The listing builds one solid part. Answer for the finished solid, in the listing's coordinates (mm). A direction names the side the tool comes from. Give positions to 0.01 mm unless a question says otherwise; leave off trailing zeros. Write each loop counter-clockwise with the first axis right and the second up, starting at its lowest first coordinate (ties: lowest second). Pieces come first, ordered by that corner, then holes. Notation, with made-up numbers: (-0.75, -16) - (40.25, -16) arc R17 ccw to (40.25, -5) - close; hole circle Ø10 at (82.5, 51). An arc over 180 degrees is marked (long way). Return JSON: item names as keys, results as strings.
from build123d import *

# Parameters (mm, degrees)
SKETCH1_W           = 160
SKETCH1_H           = 102
SKETCH1_W_2         = 154
SKETCH1_H_2         = 96
BOSS_EXTRUDE1_DEPTH = 40
SKETCH2_W           = 160
SKETCH2_H           = 102
BOSS_EXTRUDE2_DEPTH = 3
SKETCH3_R           = 1.5
BOSS_EXTRUDE3_DEPTH = 3


with BuildPart() as part:
    # Sketch1 → Boss-Extrude1 (new body)
    with BuildSketch(Plane(origin=(0, 0, 0), x_dir=(1, 0, 0), z_dir=(0, 1, 0))):
        with Locations((77, -48)):
            Rectangle(SKETCH1_W, SKETCH1_H)
        with Locations((77, -48)):
            Rectangle(SKETCH1_W_2, SKETCH1_H_2, mode=Mode.SUBTRACT)
    extrude(amount=BOSS_EXTRUDE1_DEPTH)

    # Sketch2 → Boss-Extrude2 (add)
    with BuildSketch(Plane.XZ):
        with Locations((77, 48)):
            Rectangle(SKETCH2_W, SKETCH2_H)
    extrude(amount=BOSS_EXTRUDE2_DEPTH)

    # Sketch3 → Boss-Extrude3 (add)
    with BuildSketch(Plane.XZ.offset(3)):
        with BuildLine():
            Line((87, 103), (87, -7))
            ThreePointArc((87, -7), (77, -17), (67, -7))
            Line((67, -7), (67, 103))
            ThreePointArc((67, 103), (77, 113), (87, 103))
        make_face()
        with Locations(Location((77, -7, 0), (0, 0, 270))):
            Circle(SKETCH3_R, mode=Mode.SUBTRACT)
        with Locations(Location((77, 103, 0), (0, 0, 270))):
            Circle(SKETCH3_R, mode=Mode.SUBTRACT)
    extrude(amount=-BOSS_EXTRUDE3_DEPTH)


solid = part.part
Item 1: For faces 4 (the face through (77, 0, -10)), 5 (the face through (76, 20, 96)), 6 (the face through (-3, 19, 47)), 7 (the face through (77, 0, 105)), determine the directions among +Z, -Z, +X, -X, +Y, -Y from which every point of the face is accessible in a straight line to the end or side of a thin tool.
Answer below:
{"face 4": "-Z, +X, -X, +Y", "face 5": "+Y", "face 6": "+Z, -Z, -X, +Y, -Y", "face 7": "+Z, +X, -X, +Y"}
Item 2: Flat-ended cylindrical pins translate along their axes: P1, Ø4, axis at x = 41.5, y = 2, coming from the +Z side; P2, Ø1.5, axis at y = -1, z = -5, coming from the -X side; P3, Ø7, axis at x = 74, z = -12.5, coming from the +Y side. Find the tip coordinate at first contact, or state that the pin passes through.
Answer below:
{"P1": "stops at z = 99", "P2": "stops at x = 67", "P3": "stops at y = 0"}
Item 3: The mould has two halves that part along X. Classify faces 1 (the face through (154, 20, 49)), 2 (the face through (76, 19, -3)), 3 (the face through (157, 19, 47)): +X half, -X half, draft (parallel to the pull), parting line (faces both ways), or undercut.
Answer below:
{"face 1": "undercut", "face 2": "draft", "face 3": "+X half"}
Item 4: Consider L1, parallel to Z at x = 77, y = -1.8; L2, parallel to X at y = -1.05, z = -7; L3, parallel to Z at x = 43.5, y = 7.5. Determine where each line is inside the solid, lowest interval first.
Answer below:
{"L1": "z = -17 to -8.5, -5.5 to 101.5, 104.5 to 113", "L2": "x = 67 to 75.5, 78.5 to 87", "L3": "z = -3 to 0, 96 to 99"}
Item 5: A cutting plane is placed at A-A on y = 6.5. Determine the outline of the cut face in (x, z).
Answer below:
{"outline": "(-3, -3) - (157, -3) - (157, 99) - (-3, 99) - close; hole (0, 0) - (154, 0) - (154, 96) - (0, 96) - close"}
Item 6: A cutting plane is placed at B-B on z = 78. Determine the outline of the cut face in (x, y), then the cut area to 3 significant figures.
Answer below:
{"outline": "(-3, -3) - (157, -3) - (157, 40) - (154, 40) - (154, 0) - (0, 0) - (0, 40) - (-3, 40) - close", "area": "720 mm²"}
Item 7: A cutting plane is placed at C-C on x = 40. Determine the outline of the cut face in (y, z).
Answer below:
{"outline": "(-3, -3) - (40, -3) - (40, 0) - (0, 0) - (0, 96) - (40, 96) - (40, 99) - (-3, 99) - close"}
